Input: part model. Units: mm. Frame: model coordinates. Give positions to 0.01 mm unless a question says otherwise; leave off trailing zeros. Answer as a JSON object with one key per item and string values.
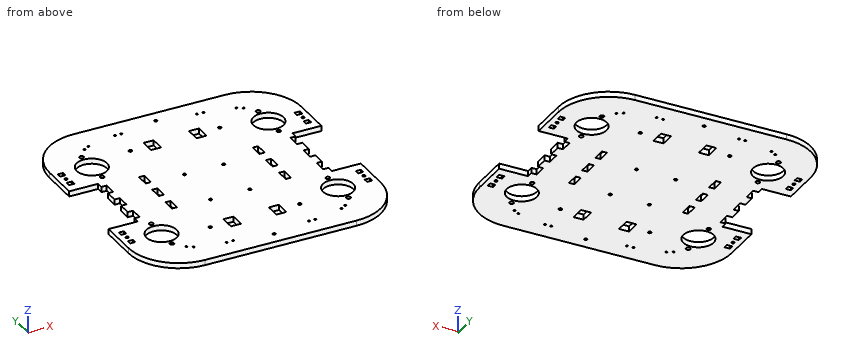
```python
from build123d import *

# Parameters (mm, degrees)
BOSS_EXTRUDE1_DEPTH = 5.334
SKETCH3_W           = 5.334
SKETCH3_H           = 12.7
CUT_EXTRUDE1_DEPTH  = 5.334
SKETCH4_R           = 1.5
CUT_EXTRUDE2_DEPTH  = 360.249845589
SKETCH5_R           = 1.651
SKETCH5_W           = 10.16
SKETCH5_H           = 14.478
CUT_EXTRUDE3_DEPTH  = 360.249845589
SKETCH6_R           = 1.5
SKETCH6_W           = 5.334
SKETCH6_H           = 4.572
CUT_EXTRUDE4_DEPTH  = 360.249845589
SKETCH7_R           = 1
SKETCH7_R_2         = 1.45
CUT_EXTRUDE5_DEPTH  = 360.249845589
SKETCH8_R           = 15.24
SKETCH8_R_2         = 2.159
CUT_EXTRUDE6_DEPTH  = 360.249845589


with BuildPart() as part:
    # Sketch1 → Boss-Extrude1 (new body)
    with BuildSketch(Plane.XY):
        with BuildLine():
            Line((50.8, 0), (203.2, 0))
            ThreePointArc((203.2, 0), (239.121024484, 14.878975516), (254, 50.8))
            Line((254, 50.8), (254, 203.2))
            ThreePointArc((254, 203.2), (239.121024484, 239.121024484), (203.2, 254))
            Line((203.2, 254), (50.8, 254))
            ThreePointArc((50.8, 254), (14.878975516, 239.121024484), (0, 203.2))
            Line((0, 203.2), (0, 50.8))
            ThreePointArc((0, 50.8), (14.878975516, 14.878975516), (50.8, 0))
        make_face()
    extrude(amount=BOSS_EXTRUDE1_DEPTH)

    # Sketch3 → Cut-Extrude1 (cut)
    with BuildSketch(Plane.XY.offset(5.334)):
        Polygon((29.21, 95.25), (29.21, 88.9), (0, 88.9), (0, 165.1), (29.21, 165.1), (29.21, 158.75), (34.544, 158.75), (34.544, 146.05), (29.21, 146.05), (29.21, 133.35), (34.544, 133.35), (34.544, 120.65), (29.21, 120.65), (29.21, 107.95), (34.544, 107.95), (34.544, 95.25), align=None)
        Polygon((224.79, 133.35), (219.456, 133.35), (219.456, 120.65), (224.79, 120.65), (224.79, 107.95), (219.456, 107.95), (219.456, 95.25), (224.79, 95.25), (224.79, 88.9), (254, 88.9), (254, 165.1), (224.79, 165.1), (224.79, 158.75), (219.456, 158.75), (219.456, 146.05), (224.79, 146.05), align=None)
        with Locations((69.723, 127)):
            Rectangle(SKETCH3_W, SKETCH3_H)
        with Locations((69.723, 152.4)):
            Rectangle(SKETCH3_W, SKETCH3_H)
        with Locations((69.723, 101.6)):
            Rectangle(SKETCH3_W, SKETCH3_H)
        with Locations((184.277, 152.4)):
            Rectangle(SKETCH3_W, SKETCH3_H)
        with Locations((184.277, 127)):
            Rectangle(SKETCH3_W, SKETCH3_H)
        with Locations((184.277, 101.6)):
            Rectangle(SKETCH3_W, SKETCH3_H)
    extrude(amount=-CUT_EXTRUDE1_DEPTH, mode=Mode.SUBTRACT)

    # Sketch4 → Cut-Extrude2 (cut, through all)
    with BuildSketch(Plane.XY.offset(5.334)):
        with Locations((105.213395979, 93.678)):
            Circle(SKETCH4_R)
        with Locations(Location((144.679395979, 93.678, 0), (0, 0, 180))):
            Circle(SKETCH4_R)
        with Locations((144.679395979, 144.32)):
            Circle(SKETCH4_R)
        with Locations(Location((105.213395979, 144.32, 0), (0, 0, 180))):
            Circle(SKETCH4_R)
    extrude(amount=-CUT_EXTRUDE2_DEPTH, mode=Mode.SUBTRACT)

    # Sketch5 → Cut-Extrude3 (cut, through all)
    with BuildSketch(Plane.XY.offset(5.334)):
        with Locations((82.042, 204.089)):
            Circle(SKETCH5_R)
        with Locations((104.14, 204.089)):
            Rectangle(SKETCH5_W, SKETCH5_H)
        with Locations((149.86, 204.089)):
            Rectangle(SKETCH5_W, SKETCH5_H)
        with Locations((171.958, 204.089)):
            Circle(SKETCH5_R)
        with Locations((82.042, 49.911)):
            Circle(SKETCH5_R)
        with Locations((104.14, 49.911)):
            Rectangle(SKETCH5_W, SKETCH5_H)
        with Locations((149.86, 49.911)):
            Rectangle(SKETCH5_W, SKETCH5_H)
        with Locations(Location((171.958, 49.911, 0), (0, 0, 180))):
            Circle(SKETCH5_R)
    extrude(amount=-CUT_EXTRUDE3_DEPTH, mode=Mode.SUBTRACT)

    # Sketch6 → Cut-Extrude4 (cut, through all)
    with BuildSketch(Plane.XY.offset(5.334)):
        with Locations((7.747, 185.928)):
            Circle(SKETCH6_R)
        with Locations(Location((246.253, 185.928, 0), (0, 0, 180))):
            Circle(SKETCH6_R)
        with Locations((246.253, 68.072)):
            Circle(SKETCH6_R)
        with Locations(Location((7.747, 68.072, 0), (0, 0, 180))):
            Circle(SKETCH6_R)
        with Locations((7.747, 194.564)):
            Rectangle(SKETCH6_W, SKETCH6_H)
        with Locations((7.747, 177.292)):
            Rectangle(SKETCH6_W, SKETCH6_H)
        with Locations((246.253, 177.292)):
            Rectangle(SKETCH6_W, SKETCH6_H)
        with Locations((246.253, 194.564)):
            Rectangle(SKETCH6_W, SKETCH6_H)
        with Locations((246.253, 59.436)):
            Rectangle(SKETCH6_W, SKETCH6_H)
        with Locations((246.253, 76.708)):
            Rectangle(SKETCH6_W, SKETCH6_H)
        with Locations((7.747, 76.708)):
            Rectangle(SKETCH6_W, SKETCH6_H)
        with Locations((7.747, 59.436)):
            Rectangle(SKETCH6_W, SKETCH6_H)
    extrude(amount=-CUT_EXTRUDE4_DEPTH, mode=Mode.SUBTRACT)

    # Sketch7 → Cut-Extrude5 (cut, through all)
    with BuildSketch(Plane.XY.offset(5.334)):
        with Locations((82.4, 19.05)):
            Circle(SKETCH7_R)
        with Locations((88.9, 19.05)):
            Circle(SKETCH7_R)
        with Locations(Location((165.1, 19.05, 0), (0, 0, 180))):
            Circle(SKETCH7_R)
        with Locations(Location((171.6, 19.05, 0), (0, 0, 180))):
            Circle(SKETCH7_R)
        with Locations((171.6, 234.95)):
            Circle(SKETCH7_R)
        with Locations((165.1, 234.95)):
            Circle(SKETCH7_R)
        with Locations(Location((88.9, 234.95, 0), (0, 0, 180))):
            Circle(SKETCH7_R)
        with Locations(Location((82.4, 234.95, 0), (0, 0, 180))):
            Circle(SKETCH7_R)
        with Locations((127, 12.7)):
            Circle(SKETCH7_R_2)
        with Locations(Location((127, 241.3, 0), (0, 0, 180))):
            Circle(SKETCH7_R_2)
        with Locations((52.518273092, 25.4)):
            Circle(SKETCH7_R)
        with Locations((46.99, 28.818800465)):
            Circle(SKETCH7_R)
        with Locations(Location((207.01, 28.818800465, 0), (0, 0, 180))):
            Circle(SKETCH7_R)
        with Locations(Location((201.481726908, 25.4, 0), (0, 0, 180))):
            Circle(SKETCH7_R)
        with Locations((201.481726908, 228.6)):
            Circle(SKETCH7_R)
        with Locations((207.01, 225.181199535)):
            Circle(SKETCH7_R)
        with Locations(Location((46.99, 225.181199535, 0), (0, 0, 180))):
            Circle(SKETCH7_R)
        with Locations(Location((52.518273092, 228.6, 0), (0, 0, 180))):
            Circle(SKETCH7_R)
    extrude(amount=-CUT_EXTRUDE5_DEPTH, mode=Mode.SUBTRACT)

    # Sketch8 → Cut-Extrude6 (cut, through all)
    with BuildSketch(Plane.XY.offset(5.334)):
        with Locations((38.1, 59.69)):
            Circle(SKETCH8_R)
        with Locations((38.1, 39.751)):
            Circle(SKETCH8_R_2)
        with Locations((38.1, 79.629)):
            Circle(SKETCH8_R_2)
        with Locations(Location((215.9, 79.629, 0), (0, 0, 180))):
            Circle(SKETCH8_R_2)
        with Locations(Location((215.9, 39.751, 0), (0, 0, 180))):
            Circle(SKETCH8_R_2)
        with Locations(Location((215.9, 59.69, 0), (0, 0, 180))):
            Circle(SKETCH8_R)
        with Locations((215.9, 194.31)):
            Circle(SKETCH8_R)
        with Locations((215.9, 214.249)):
            Circle(SKETCH8_R_2)
        with Locations((215.9, 174.371)):
            Circle(SKETCH8_R_2)
        with Locations(Location((38.1, 174.371, 0), (0, 0, 180))):
            Circle(SKETCH8_R_2)
        with Locations(Location((38.1, 214.249, 0), (0, 0, 180))):
            Circle(SKETCH8_R_2)
        with Locations(Location((38.1, 194.31, 0), (0, 0, 180))):
            Circle(SKETCH8_R)
    extrude(amount=-CUT_EXTRUDE6_DEPTH, mode=Mode.SUBTRACT)


solid = part.part
```
Q1. Section A-A, the plane z = 1.5. Give the number of separate pieces and of enclosed holes in the cut face, then the cut area to 3 significant figures.
Evaluation:
{"separate pieces": "1", "enclosed holes": "60", "area": "53,100 mm2"}
Q2. Pin query (flat end, axial travel): pin 1 (1.7 mm diameter, centred on x = 127, y = 241.3, fed in from -Z); pin 2 (1.6 mm diameter, centred on y = 101.5, z = 1.5, fed in from +X); pin 3 (1.6 mm diameter, centred on x = 221, z = 3, fed in from +Y); pin 4 (4 mm diameter, centred on x = 98, y = 129, fed in from -Z). Return the tip coordinate at first contact, or that it passes through.
Evaluation:
{"pin 1": "passes through", "pin 2": "stops at x = 219.46", "pin 3": "stops at y = 251.07", "pin 4": "stops at z = 0"}
Q3. Ray query, line 1 along Y through (x, z) = (234, 1.15); line 2 along Y through (x, z) = (101, 2.95); line 3 along X through (y, z) = (174.5, 4.3). Return the intervals inside material, ascending.
Evaluation:
{"line 1": "y = 10.4 to 88.9, 165.1 to 243.6", "line 2": "y = 0 to 42.67, 57.15 to 196.85, 211.33 to 254", "line 3": "x = 0 to 35.94, 40.26 to 213.74, 218.06 to 254"}
